Input: dimensioned drawing with shaded views. Units: mm. Origin: part minimum x, y, z. Give positions to 0.01 mm unless a question says otherwise; leave off trailing zeros. Write each loop counter-clockwise with the first axis right and the second up, starting at its lowest first coordinate (ties: lowest second). Pieces come first, ordered by that corner, then holes. Notation, with made-up numbers: (37.25, 32) -> (69.25, 32) arc R20 cw to (69.25, 40) -> close; hole circle Ø3 at (73.25, 88.25). An arc over 180 degrees is marked (long way). Answer as a JSON object with one key per item and string values. Group by question number.
(1) Material intervals for probe 1 along Z at (x, y) = (39.5, 5.5); probe 2 along X at (y, z) = (6, 62.5); probe 3 along Z at (x, y) = (41.5, 3), sorted ascending.
(2) Section query C-C on x = 5. Output: boundary loops of the cut face in (y, z).
(3) Contact query for flat-ended pins moving along their axis: pin 1 Ø2 at (y, z) = (4, 4.5) entering from +X; pin 2 Ø3 at (y, z) = (4, 74.5) entering from +X; pin 3 Ø1 at (x, y) = (40.5, 1) entering from +Z; pin 4 Ø1 at (x, y) = (14.5, 1.5) entering from -Z. Output: stop coordinate, or through.
(4) Section query D-D on z = 42.5. Output: boundary loops of the cut face in (x, y).
(5) Section query A-A on x = 42.5. Output: boundary loops of the cut face in (y, z), plus the area to 4 significant figures.
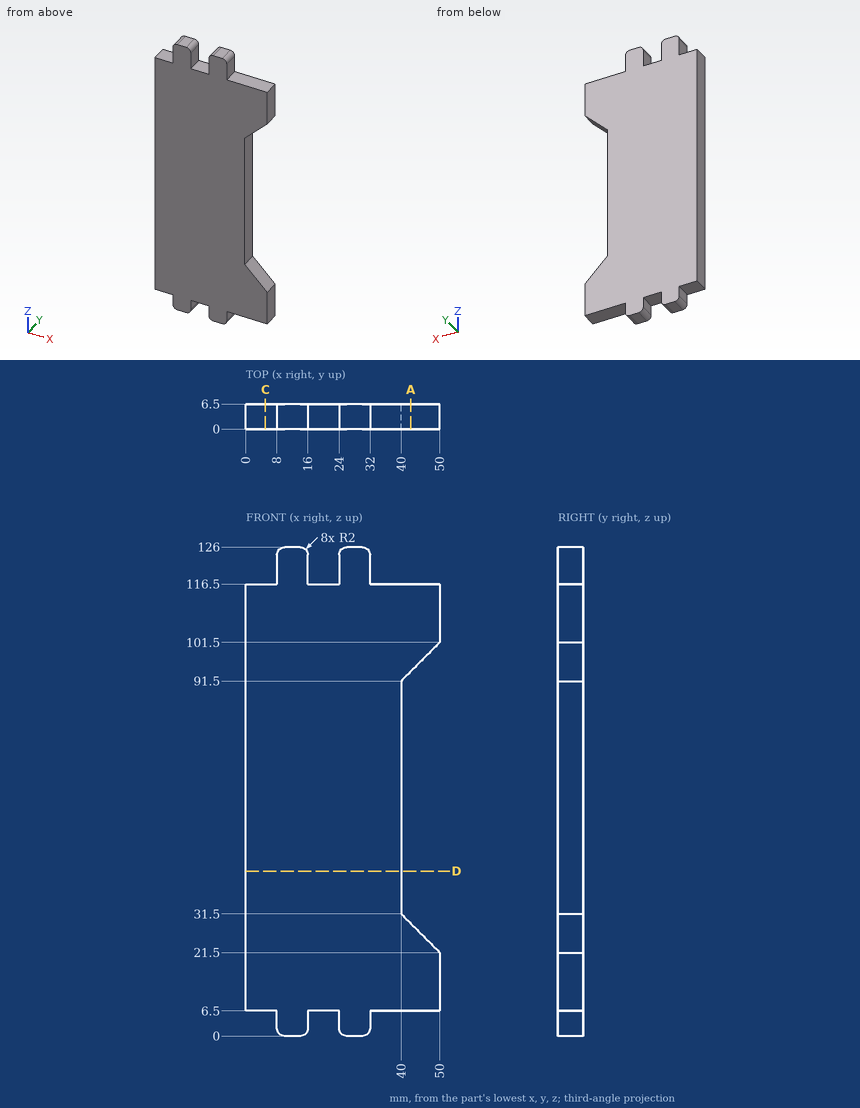
Answer list:
{
 "1": {"probe 1": "6.5 to 116.5", "probe 2": "0 to 40", "probe 3": "6.5 to 30, 93 to 116.5"},
 "2": {"outline": "(0, 6.5) -> (6.5, 6.5) -> (6.5, 116.5) -> (0, 116.5) -> close"},
 "3": {"pin 1": "x = 32", "pin 2": "x = 40", "pin 3": "z = 116.5", "pin 4": "z = 0"},
 "4": {"outline": "(0, 0) -> (40, 0) -> (40, 6.5) -> (0, 6.5) -> close"},
 "5": {"outline": "(0, 6.5) -> (6.5, 6.5) -> (6.5, 29) -> (0, 29) -> close; (0, 94) -> (6.5, 94) -> (6.5, 116.5) -> (0, 116.5) -> close", "area": "292.5 mm2"}
}
